For this review, take the finished solid that the model builds, in its own axes (mm). A direction names the side the tool comes from. Give positions to 0.01 mm unless a question says otherwise; leave off trailing zeros. Loops run counter-clockwise (first coordinate to the right, second up) from the corner with the lowest first, then second, coordinate; pieces in that order, holes last.
```python
from build123d import *

# Parameters (mm, degrees)
SKETCH1_W           = 25.4
SKETCH1_H           = 50.8
BOSS_EXTRUDE1_DEPTH = 406.4
SHELL1_T            = -3.175
SKETCH2_R           = 12.7
SKETCH2_R_2         = 2.4892
CUT_EXTRUDE1_DEPTH  = 411.349558304


with BuildPart() as part:
    # Sketch1 → Boss-Extrude1 (new, symmetric)
    with BuildSketch(Plane(origin=(0, 0, 0), x_dir=(1, 0, 0), z_dir=(0, 1, 0))):
        with Locations((12.7, 25.4)):
            Rectangle(SKETCH1_W, SKETCH1_H)
    extrude(amount=BOSS_EXTRUDE1_DEPTH, both=True)

    # Shell1
    shell1_openings = [part.faces().sort_by_distance(p)[0] for p in [
        (12.7, 406.4, -25.4),
        (12.7, -406.4, -25.4),
    ]]
    offset(amount=SHELL1_T, openings=shell1_openings, kind=Kind.INTERSECTION)

    # Sketch2 → Cut-Extrude1 (cut, through all)
    with BuildSketch(Plane(origin=(25.4, 0, 0), x_dir=(0, 0, -1), z_dir=(1, 0, 0))):
        with Locations((25.4, 374.65)):
            Circle(SKETCH2_R)
        with Locations((25.4, -374.65)):
            Circle(SKETCH2_R)
        with Locations((25.4, 298.45)):
            Circle(SKETCH2_R_2)
    extrude(amount=-CUT_EXTRUDE1_DEPTH, mode=Mode.SUBTRACT)


solid = part.part
```
Q1. Machinability: for faces 5 (the flat face through (22.225, 6, -25)), 6 (the cylindrical face through (23.83, -387.05, -22.65)), which of the approach directions +Z, -Z, +X, -X, +Y, -Y give a long, thin tool a straight path to every point of the face, cutting with its end or side? Answer none if there is none.
Answers:
face 5: +Y, -Y
face 6: +X, -X
Q2. Consider section B-B on x = 15. Give the boundary of the cut face in (y, z) (3 decimals).
Answers:
outline: (-406.4, -50.8) - (406.4, -50.8) - (406.4, -47.625) - (-406.4, -47.625) - close; (-406.4, -3.175) - (406.4, -3.175) - (406.4, 0) - (-406.4, 0) - close
Q3. Consider section A-A on y = -374.65. Give the boundary of the cut face in (x, z) (3 decimals), plus the area to 3 significant figures.
Answers:
outline: (0, -50.8) - (25.4, -50.8) - (25.4, -38.1) - (22.225, -38.1) - (22.225, -47.625) - (3.175, -47.625) - (3.175, -38.1) - (0, -38.1) - close; (0, -12.7) - (3.175, -12.7) - (3.175, -3.175) - (22.225, -3.175) - (22.225, -12.7) - (25.4, -12.7) - (25.4, 0) - (0, 0) - close
area: 282 mm2
Q4. For probe 1 along Y at (x, z) = (23.8, -25.4); probe 2 along Z at (x, y) = (12, 120.5) (3 decimals); probe 3 along X at (y, z) = (260.5, -30) (3 decimals), list the stretches that pass through material, from the lowest coordinate up.
Answers:
probe 1: y = -406.4 to -387.35, -361.95 to 295.96, 300.94 to 361.95, 387.35 to 406.4
probe 2: z = -50.8 to -47.625, -3.175 to 0
probe 3: x = 0 to 3.175, 22.225 to 25.4
Q5. Mouldability with a two-part tool opening along Y and no side actions: class faces 1 (the cylindrical face through (1.61, 383.233, -16.04)), 2 (the flat face through (13, 6, -3.175)), 3 (the flat face through (2, 406.4, -24)), 4 (the cylindrical face through (23.835, 383.233, -16.04)) as +Y half, -Y half, draft (parallel to the pull), parting line (faces both ways), or undercut.
Answers:
face 1: undercut
face 2: draft
face 3: +Y half
face 4: undercut
Q6. Consider section C-C on y = 350. Give the boundary of the cut face in (x, z) (3 decimals), plus the area to 3 significant figures.
Answers:
outline: (0, -50.8) - (25.4, -50.8) - (25.4, 0) - (0, 0) - close; hole (3.175, -47.625) - (22.225, -47.625) - (22.225, -3.175) - (3.175, -3.175) - close
area: 444 mm2
